from build123d import *

# Parameters (mm, degrees)
SKETCH1_W           = 15
SKETCH1_H           = 15
SKETCH1_W_2         = 11
SKETCH1_H_2         = 11
BOSS_EXTRUDE1_DEPTH = 400
SKETCH2_R           = 1.6
CUT_EXTRUDE1_DEPTH  = 401.562105047
SKETCH3_R           = 1.6
CUT_EXTRUDE2_DEPTH  = 401.562105047


with BuildPart() as part:
    # Sketch1 → Boss-Extrude1 (new body)
    with BuildSketch(Plane(origin=(0, 0, 0), x_dir=(1, 0, 0), z_dir=(0, 1, 0))):
        with Locations((7.5, 7.5)):
            Rectangle(SKETCH1_W, SKETCH1_H)
        with Locations((7.5, 7.5)):
            Rectangle(SKETCH1_W_2, SKETCH1_H_2, mode=Mode.SUBTRACT)
    extrude(amount=BOSS_EXTRUDE1_DEPTH)

    # Sketch2 → Cut-Extrude1 (cut, through all)
    with BuildSketch(Plane.XY):
        with Locations((7.5, 9.6)):
            Circle(SKETCH2_R)
        with Locations((7.5, 39.6)):
            Circle(SKETCH2_R)
        with Locations((7.5, 56.7)):
            Circle(SKETCH2_R)
        with Locations((7.5, 81.7)):
            Circle(SKETCH2_R)
        with Locations((7.5, 106.7)):
            Circle(SKETCH2_R)
        with Locations((7.5, 131.7)):
            Circle(SKETCH2_R)
        with Locations((7.5, 156.7)):
            Circle(SKETCH2_R)
        with Locations((7.5, 243.3)):
            Circle(SKETCH2_R)
        with Locations((7.5, 268.3)):
            Circle(SKETCH2_R)
        with Locations((7.5, 293.3)):
            Circle(SKETCH2_R)
        with Locations((7.5, 318.3)):
            Circle(SKETCH2_R)
        with Locations((7.5, 343.3)):
            Circle(SKETCH2_R)
        with Locations((7.5, 360.4)):
            Circle(SKETCH2_R)
        with Locations((7.5, 390.4)):
            Circle(SKETCH2_R)
    extrude(amount=-CUT_EXTRUDE1_DEPTH, mode=Mode.SUBTRACT)

    # Sketch3 → Cut-Extrude2 (cut, through all)
    with BuildSketch(Plane(origin=(15, 0, 0), x_dir=(0, 0, -1), z_dir=(1, 0, 0))):
        with Locations((7.5, 143)):
            Circle(SKETCH3_R)
        with Locations((7.5, 167)):
            Circle(SKETCH3_R)
        with Locations((7.5, 233)):
            Circle(SKETCH3_R)
        with Locations((7.5, 257)):
            Circle(SKETCH3_R)
    extrude(amount=-CUT_EXTRUDE2_DEPTH, mode=Mode.SUBTRACT)


solid = part.part
Could you check a few things on this model? Use its own coordinates, in mm. A direction names the side the tool comes from. Coordinates: 2 decimals unless noted, no trailing zeros. Loops run counter-clockwise (first coordinate to the right, second up) from the corner with the lowest first, then second, coordinate; pieces in that order, holes last.
1. For P1, Ø1.9, axis at x = 7.5, y = 390.4, coming from the -Z side, with a flat end and sliding along its axis, tell me the tip position at first contact or that it passes through.
2. We'd pull the mould along X, two halves only. Please class faces 1 (the face through (2, 197, -7)), 2 (the face through (13, 197, -7)), 3 (the face through (14, 400, -8)), 4 (the face through (0, 197, -7)): released by +X, released by -X, zero draft, split by the parting line, or undercut.
3. Imagine slicing it at A-A (y = 28.5). Please give me the cut outline in (x, z), and give its area (3 significant figures).
4. I need wall thicknesses on L1, parallel to Y at x = 0.75, z = -7.5; L2, parallel to X at y = 126.5, z = -4; L3, parallel to Z at x = 7.25, y = 331. Which ranges of each line are inside material? Lowest first, please.
5. For faces 5 (the face through (7, 197, -13)), 6 (the face through (15, 197, -7)), which set-ups out of +Z, -Z, +X, -X, +Y, -Y let a thin tool reach every point of the face, with its end or its side?
Computed values:
1. P1: passes through
2. face 1: undercut
2. face 2: undercut
2. face 3: zero draft
2. face 4: released by -X
3. outline: (0, -15) - (15, -15) - (15, 0) - (0, 0) - close; hole (2, -13) - (13, -13) - (13, -2) - (2, -2) - close
3. area: 104 mm2
4. L1: y = 0 to 141.4, 144.6 to 165.4, 168.6 to 231.4, 234.6 to 255.4, 258.6 to 400
4. L2: x = 0 to 2, 13 to 15
4. L3: z = -15 to -13, -2 to 0
5. face 5: +Y, -Y
5. face 6: +Z, -Z, +X, +Y, -Y
